Study the drawing (mm; zero at the part's minimum x, y, z) and answer. Give positions to 0.01 mm unless a question says otherwise; leave off trailing zeros. Loops run counter-clockwise (first coordinate to the right, second up) from the corner with the lowest first, then second, coordinate; pieces in that order, holes last. Notation, with made-up numbers: (22.25, 2) - (58.25, 2) arc R13 ccw to (58.25, 20) - close; hole circle Ø4 at (64, 55.25). An arc over 180 degrees is marked (long way). Use one line per item in the form item = value. Start each with the question number.
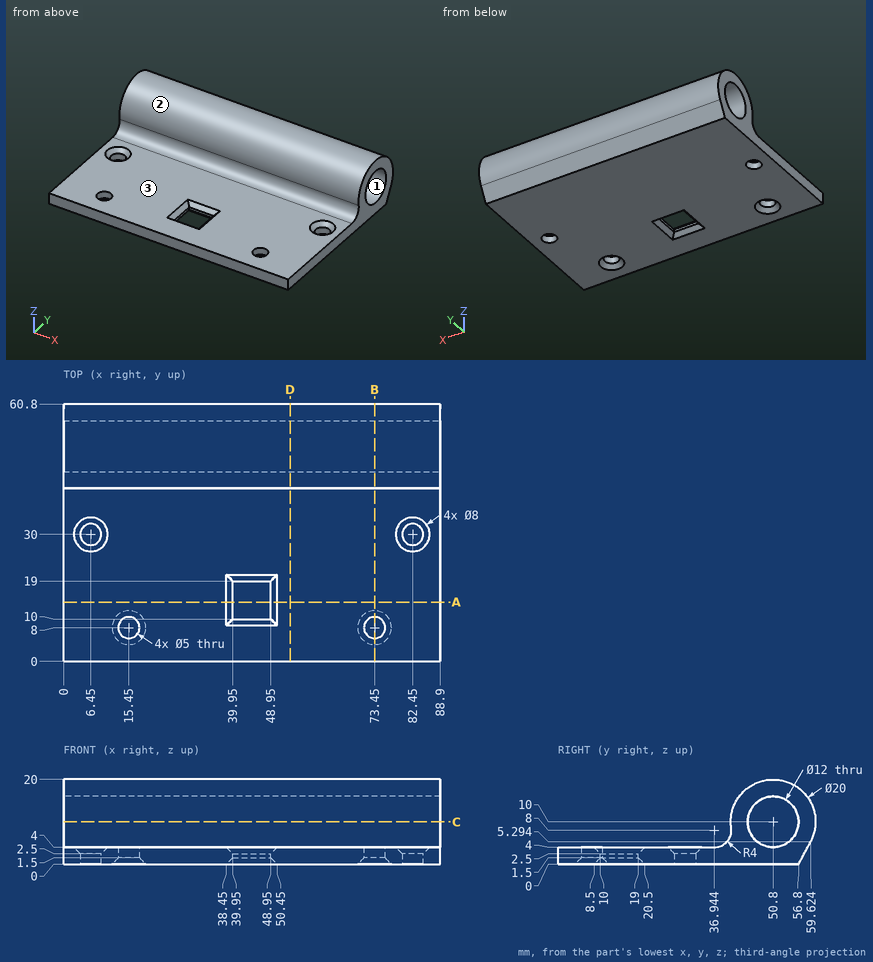
1) Flat-ended cylindrical pins translate along their axes: pin 1 Ø1.5 at (x, y) = (46, 48) entering from +Z; pin 2 Ø6.5 at (x, y) = (73.45, 8) entering from -Z; pin 3 Ø0.5 at (x, z) = (44, 2) entering from +Y. Find the tip coordinate at first contact, or state that the pin passes through.
2) A cutting plane is placed at D-D (x = 53.5). Give the vertices of the cut face in (y, z) (1 decimal).
3) A cutting plane is placed at A-A (y = 14). Give the vertices of the cut face in (x, z), plus the area to 3 significant figures.
4) Find the intervals of material crossed by probe 1 along Z at (x, y) = (57, 50.8); probe 2 along X at (y, z) = (30, 3.5); probe 3 along Z at (x, y) = (46.5, 8), in increasing order.
5) A cutting plane is placed at C-C (z = 10). Give the vertices of the cut face in (x, y).
6) A cutting plane is placed at B-B (x = 73.45). Give the vertices of the cut face in (y, z) (1 decimal).
7) Determine the mould class of the marked faces 1, 2 and 3 for opening direction Y: released by +Y, released by -Y, zero draft, split by the parting line, or undercut.
Answer sheet:
q1.pin_1 = 19.79
q1.pin_2 = 0.75
q1.pin_3 = 58
q2.outline = (0, 0) - (56.8, 0) - (59.6, 5.3) arc R10 ccw (long way) to (40.9, 8.6) arc R4 cw to (36.9, 4) - (0, 4) - close; hole circle Ø12 at (50.8, 10)
q3.outline = (0, 0) - (38.45, 0) - (39.95, 1.5) - (39.95, 2.5) - (38.45, 4) - (0, 4) - close; (48.95, 1.5) - (50.45, 0) - (88.9, 0) - (88.9, 4) - (50.45, 4) - (48.95, 2.5) - close
q3.area = 315 mm²
q4.probe_1 = 0 to 4, 16 to 20
q4.probe_2 = 0 to 2.95, 9.95 to 78.95, 85.95 to 88.9
q4.probe_3 = 0 to 4
q5.outline = (0, 40.8) - (88.9, 40.8) - (88.9, 44.8) - (0, 44.8) - close; (0, 56.8) - (88.9, 56.8) - (88.9, 60.8) - (0, 60.8) - close
q6.outline = (0, 0) - (4, 0) - (5.5, 1.5) - (5.5, 4) - (0, 4) - close; (10.5, 1.5) - (12, 0) - (56.8, 0) - (59.6, 5.3) arc R10 ccw (long way) to (40.9, 8.6) arc R4 cw to (36.9, 4) - (10.5, 4) - close; hole circle Ø12 at (50.8, 10)
q7.face_1 = undercut
q7.face_2 = split by the parting line
q7.face_3 = zero draft
